Source: CAD feature listing. Evaluate the final solid. Frame: model axes, mm. A direction names the side the tool comes from. Coordinates: 2 decimals unless noted, no trailing zeros. Write each loop counter-clockwise with the first axis right and the second up, starting at its lowest first coordinate (ties: lowest second). Pieces come first, ordered by that corner, then holes. Notation, with made-up numbers: (9.5, 83.5) - (21.5, 83.5) arc R14 cw to (21.5, 100.5) - close; hole circle Ø5 at (78, -30.75). An arc over 180 degrees is marked (long way). One line per question, with ' | ' between items. Start each with the question number.
Q1. Cut plane D-D, the plane x = 6. Return loops of the section in (y, z), plus the area to 3 significant figures.
Q2. Access query for faces 1 (the face through (11.41, -3, 0)), 2 (the face through (0, 0, 0)). Directions: +Z, -Z, +X, -X, +Y, -Y. A direction counts if a zero-diameter tool reaches every point of the face in a straight line with its end or side. Return the directions, or none.
Q3. Line query: line 1 (Z direction, x = -7.75, y = -5.05); line 2 (X direction, y = -3.6, z = 2); line 3 (Y direction, x = -2.75, z = 0.5). Output: solid intervals per line, ascending.
Q4. Cut plane B-B, the plane y = -2.85. Return loops of the section in (x, z) (3 decimals), plus the area to 3 significant figures.
Q5. Cut plane C-C, the plane z = -4. Return loops of the section in (x, y).
Q6. Cut plane A-A, the plane x = -11. Return loops of the section in (y, z), plus the area to 3 significant figures.
Q7. Draft query along X for faces 3 (the face through (0, -3, -6.2)), 4 (the face through (12.54, -3, 0)), 5 (the face through (-11.41, -3, 0)), 6 (the face through (-1, -5.6, -6.5)). Return one class per face: +X half, -X half, draft (parallel to the pull), parting line (faces both ways), or undercut.
Q8. Contact query for flat-ended pins moving along their axis: P1, Ø6, axis at x = 6.5, z = -3, coming from the +Y side; P2, Ø3, axis at x = 6, z = -2.5, coming from the -Y side. Output: stop coordinate, or through.
```python
from build123d import *

# Parameters (mm, degrees)
F0_W     = 25.08
F0_H     = 14.66
F1_DEPTH = 5.6
F2_DEPTH = 1.13


with BuildPart() as f1:
    # F0 (on Front) → F1 (new body)
    with BuildSketch(Plane.XZ):
        Rectangle(F0_W, F0_H)
        with BuildLine():
            Line((-10.2486038969, 6.2), (10.2486038969, 6.2))
            ThreePointArc((10.2486038969, 6.2), (11.1639249137, 6.4514186323), (11.71, 5.675))
            ThreePointArc((11.71, 5.675), (11.6312405778, 5.323218818), (11.41, 5.0386038969))
            Line((11.41, 5.0386038969), (11.41, -5.0386038969))
            ThreePointArc((11.41, -5.0386038969), (11.6312405778, -5.323218818), (11.71, -5.675))
            ThreePointArc((11.71, -5.675), (11.1639249137, -6.4514186323), (10.2486038969, -6.2))
            Line((10.2486038969, -6.2), (-10.2486038969, -6.2))
            ThreePointArc((-10.2486038969, -6.2), (-11.4683630945, -6.2583630945), (-11.41, -5.0386038969))
            Line((-11.41, -5.0386038969), (-11.41, 5.0386038969))
            ThreePointArc((-11.41, 5.0386038969), (-11.4683630945, 6.2583630945), (-10.2486038969, 6.2))
        make_face(mode=Mode.SUBTRACT)
    extrude(amount=F1_DEPTH)

    # F0 (on Front) → F2 (join)
    with BuildSketch(Plane.XZ):
        Rectangle(F0_W, F0_H)
        with BuildLine():
            Line((-10.2486038969, 6.2), (10.2486038969, 6.2))
            ThreePointArc((10.2486038969, 6.2), (11.1639249137, 6.4514186323), (11.71, 5.675))
            ThreePointArc((11.71, 5.675), (11.6312405778, 5.323218818), (11.41, 5.0386038969))
            Line((11.41, 5.0386038969), (11.41, -5.0386038969))
            ThreePointArc((11.41, -5.0386038969), (11.6312405778, -5.323218818), (11.71, -5.675))
            ThreePointArc((11.71, -5.675), (11.1639249137, -6.4514186323), (10.2486038969, -6.2))
            Line((10.2486038969, -6.2), (-10.2486038969, -6.2))
            ThreePointArc((-10.2486038969, -6.2), (-11.4683630945, -6.2583630945), (-11.41, -5.0386038969))
            Line((-11.41, -5.0386038969), (-11.41, 5.0386038969))
            ThreePointArc((-11.41, 5.0386038969), (-11.4683630945, 6.2583630945), (-10.2486038969, 6.2))
        make_face(mode=Mode.SUBTRACT)
        with BuildLine():
            ThreePointArc((11.41, 5.0386038969), (10.3016369055, 5.0916369055), (10.2486038969, 6.2))
            Line((10.2486038969, 6.2), (-10.2486038969, 6.2))
            ThreePointArc((-10.2486038969, 6.2), (-10.1085813677, 5.9539249137), (-10.06, 5.675))
            ThreePointArc((-10.06, 5.675), (-10.533218818, 4.9287594222), (-11.41, 5.0386038969))
            Line((-11.41, 5.0386038969), (-11.41, -5.0386038969))
            ThreePointArc((-11.41, -5.0386038969), (-10.533218818, -4.9287594222), (-10.06, -5.675))
            ThreePointArc((-10.06, -5.675), (-10.1085813677, -5.9539249137), (-10.2486038969, -6.2))
            Line((-10.2486038969, -6.2), (10.2486038969, -6.2))
            ThreePointArc((10.2486038969, -6.2), (10.3016369055, -5.0916369055), (11.41, -5.0386038969))
            Line((11.41, -5.0386038969), (11.41, 5.0386038969))
        make_face()
    extrude(amount=F2_DEPTH)


solid = f1.part
```
Reply:
1) outline: (-5.6, -7.33) - (0, -7.33) - (0, 7.33) - (-5.6, 7.33) - (-5.6, 6.2) - (-1.13, 6.2) - (-1.13, -6.2) - (-5.6, -6.2) - close | area: 26.7 mm^2
2) face 1: -Y | face 2: +Z, -Z, +X, -X, +Y
3) line 1: z = -7.33 to -6.2, 6.2 to 7.33 | line 2: x = -12.54 to -11.41, 11.41 to 12.54 | line 3: y = -1.13 to 0
4) outline: (-12.54, -7.33) - (12.54, -7.33) - (12.54, 7.33) - (-12.54, 7.33) - close; hole (-11.41, -5.039) arc R0.825 ccw (long way) to (-10.249, -6.2) - (10.249, -6.2) arc R0.825 ccw (long way) to (11.41, -5.039) - (11.41, 5.039) arc R0.825 ccw (long way) to (10.249, 6.2) - (-10.249, 6.2) arc R0.825 ccw (long way) to (-11.41, 5.039) - close | area: 82.6 mm^2
5) outline: (-12.54, -5.6) - (-11.41, -5.6) - (-11.41, -1.13) - (11.41, -1.13) - (11.41, -5.6) - (12.54, -5.6) - (12.54, 0) - (-12.54, 0) - close
6) outline: (-5.6, -7.33) - (0, -7.33) - (0, -6.49) - (-5.6, -6.49) - close; (-5.6, 6.49) - (0, 6.49) - (0, 7.33) - (-5.6, 7.33) - close; (-1.13, -4.86) - (0, -4.86) - (0, 4.86) - (-1.13, 4.86) - close | area: 20.4 mm^2
7) face 3: undercut | face 4: +X half | face 5: undercut | face 6: draft
8) P1: stops at y = 0 | P2: stops at y = -1.13
